Work out the finished part from the listing and answer in its coordinate system (mm). A direction names the side the tool comes from. Coordinates: 2 decimals unless noted, no trailing zeros. Write each loop counter-clockwise with the first axis right and the second up, starting at its lowest first coordinate (ties: lowest second). Pieces come first, ordered by that corner, then holes. Notation, with made-up numbers: (21, -9.5) - (72, -9.5) arc R14 cw to (72, 16.5) - close; hole circle Ø5 at (18, -17). An arc over 180 degrees is marked (long way). One line per item, written item: value.
Autodesk Inventor part; units mm, degrees
ref_plane "YZ Plane" through (0, 0, 0) normal (1, 0, 0) x (0, 1, 0)
ref_plane "XZ Plane" through (0, 0, 0) normal (0, 1, 0) x (-1, 0, 0)
ref_plane "XY Plane" through (0, 0, 0) normal (0, 0, 1) x (1, 0, 0)
sketch "Sketch1" plane through (0, 0, 0) normal (0, 1, 0) x (-1, 0, 0)
  line L0 (0, 0) -> (-40.64, 0)
  line L1 (-40.64, 0) -> (-40.64, -33.147)
  line L2 (-40.64, -33.147) -> (0, -33.147)
  line L3 (0, -33.147) -> (0, 0)
  dimension "d0" = 40.64
  dimension "d1" = 33.147
extrude "Extrusion1" add sketch "Sketch1" along normal mid plane 19.05
sketch "Sketch2" plane through (0, -9.525, 0) normal (0, 0, 1) x (1, 0, 0)
  line L0 (0, -6.3625) -> (40.64, -6.3625)
  line L1 (40.64, -6.3625) -> (40.64, 12.6875)
  line L2 (40.64, 12.6875) -> (0, 12.6875)
  line L3 (0, 12.6875) -> (0, -6.3625)
  point P0 (0, 9.525)
  dimension "d4" = 40.64
  dimension "d5" = 19.05
extrude "Extrusion2" add sketch "Sketch2" along normal blind 6.35
sketch "Sketch3" plane through (0, -9.525, 6.35) normal (0, 0, 1) x (1, 0, 0)
  line L0 (40.64, 12.6875) -> (0, 12.6875)
  point P0 (0, 9.525)
sketch "Sketch7" plane through (0, -9.525, 6.35) normal (0, 0, 1) x (1, 0, 0)
  point P0 (0, 9.525)
sketch "Sketch8" plane through (0, -15.8875, 0) normal (0, -1, 0) x (1, 0, 0)
  line L0 (40.64, 6.35) -> (0, 6.35)
  line L1 (40.64, 0) -> (0, 0)
  line L2 (0, 6.35) -> (40.64, 6.35)
  line L3 (40.64, 6.35) -> (40.64, 0)
  line L4 (40.64, 0) -> (0, 0)
  line L5 (0, 0) -> (0, 6.35)
extrude "Extrusion5" add sketch "Sketch8" along normal blind 6.35
sketch "Sketch9" plane through (0, 3.1625, 0) normal (0, 1, 0) x (1, 0, 0)
  line L0 (40.64, 0) -> (40.64, -6.35)
  line L1 (0, 33.147) -> (0, 0)
  line L2 (40.64, -6.35) -> (0, -6.35)
  line L3 (0, -6.35) -> (0, 0)
  line L4 (0, 0) -> (40.64, 0)
  line L5 (40.64, 0) -> (40.64, -6.35)
extrude "Extrusion6" add sketch "Sketch9" along normal blind 6.35
sketch "Sketch10" plane through (0, -9.525, 6.35) normal (0, 0, 1) x (1, 0, 0)
  line L0 (0, 9.525) -> (0, 19.05)
  circle A0 centre (20.32, 3.175) radius 15.3561
extrude "Extrusion7" add sketch "Sketch10" along normal blind 3.175
sketch "Sketch11" plane through (20.32, -6.35, 9.525) normal (0, 0, 1) x (1, 0, 0)
  circle A0 centre (0, 0) radius 9.525
  point P0 (-20.32, 6.35)
  dimension "d27" = 19.05
extrude "Extrusion8" add sketch "Sketch11" along normal blind 4.826
sketch "Sketch12" plane through (20.32, -6.35, 14.351) normal (0, 0, 1) x (1, 0, 0)
  circle A0 centre (0, 0) radius 15.3561
  point P0 (-20.32, 6.35)
extrude "Extrusion9" add sketch "Sketch12" along normal blind 11.43
sketch "Sketch13" plane through (20.32, -6.35, 25.781) normal (0, 0, 1) x (1, 0, 0)
  circle A0 centre (0, 0) radius 14.5863
  circle A1 centre (0, 0) radius 13.9111
  point P0 (-20.32, 6.35)
extrude "Extrusion10" add sketch "Sketch13" along normal blind 5.588
sketch "Sketch14" plane through (20.32, -6.35, 25.781) normal (0, 0, 1) x (1, 0, 0)
  circle A0 centre (0, 0) radius 13.5059
  point P0 (-20.32, 6.35)
extrude "Extrusion11" add sketch "Sketch14" along normal blind 5.588
thread "Thread3"
properties part number "imdreset"
Item 1: Section D-D, the plane z = 17 is taken. Determine the outline of the cut face in (x, y).
Evaluation:
outline: circle Ø30.71 at (20.32, -6.35)
Item 2: Determine the mould class of faces 1 (the face through (18.421, -20.812, 28.536)), 2 (the face through (6.422, -6.962, 28.536)), 3 (the face through (13, -13, 14.351)) for opening direction X: +X half, -X half, draft (parallel to the pull), parting line (faces both ways), or undercut.
Evaluation:
face 1: parting line
face 2: undercut
face 3: draft
Item 3: Consider probe 1 along Y at (x, z) = (20.32, 29.3); probe 2 along X at (y, z) = (-6, 29); probe 3 along Z at (x, y) = (28, -13) (3 decimals). Determine where each line is inside the solid, lowest interval first.
Evaluation:
probe 1: y = -20.94 to -20.26, -19.86 to 7.16, 7.56 to 8.24
probe 2: x = 5.74 to 6.41, 6.82 to 33.82, 34.23 to 34.9
probe 3: z = 0 to 9.525, 14.351 to 31.369
Item 4: Section A-A, the plane y = -6.35 is taken. Determine the outline of the cut face in (x, z) (3 decimals).
Evaluation:
outline: (0, -33.147) - (40.64, -33.147) - (40.64, 6.35) - (35.676, 6.35) - (35.676, 9.525) - (29.845, 9.525) - (29.845, 14.351) - (35.676, 14.351) - (35.676, 25.781) - (34.906, 25.781) - (34.906, 31.369) - (34.231, 31.369) - (34.231, 25.781) - (33.826, 25.781) - (33.826, 31.369) - (6.814, 31.369) - (6.814, 25.781) - (6.409, 25.781) - (6.409, 31.369) - (5.734, 31.369) - (5.734, 25.781) - (4.964, 25.781) - (4.964, 14.351) - (10.795, 14.351) - (10.795, 9.525) - (4.964, 9.525) - (4.964, 6.35) - (0, 6.35) - close
Item 5: Which of the six approach directions +Z, -Z, +X, -X, +Y, -Y give full straight-line access (tool end or side, diameter ignored) to faces 4 (the face through (18.26, 2.95, 11.9)), 5 (the face through (20, -6, 31.369)), 6 (the face through (21, -9.525, -16)), 7 (the face through (34, -14, 6.35))?
Evaluation:
face 4: none
face 5: +Z, +X, -X, +Y, -Y
face 6: -Z, +X, -X, -Y
face 7: +Z
Item 6: Section C-C, the plane y = 6 is taken. Determine the outline of the cut face in (x, z) (3 decimals), then the cut area to 3 significant figures.
Evaluation:
outline: (0, -33.147) - (40.64, -33.147) - (40.64, 6.35) - (29.446, 6.35) - (29.446, 9.525) - (11.194, 9.525) - (11.194, 6.35) - (0, 6.35) - close; (11.194, 14.351) - (29.446, 14.351) - (29.446, 25.781) - (28.081, 25.781) - (28.081, 31.369) - (26.723, 31.369) - (26.723, 25.781) - (25.787, 25.781) - (25.787, 31.369) - (14.853, 31.369) - (14.853, 25.781) - (13.917, 25.781) - (13.917, 31.369) - (12.559, 31.369) - (12.559, 25.781) - (11.194, 25.781) - close
area: 1,950 mm2
Item 7: Given pin 1 (10 mm diameter, centred on y = -7.5, z = 21, fed in from -X), flat-ended and moving along its own axis, determine where the tip first touches the part or whether it passes through.
Evaluation:
pin 1: stops at x = 4.96
